Read the model definition and answer for the solid it produces. Units are mm, in the model's axes. Face numbers are marked on the shaded views. A direction names the side the tool comes from. Coordinates: 2 decimals unless noted, no trailing zeros. Order: outer loops, then holes, each group sorted by start corner. A loop starts at its lowest first (then second) coordinate and runs counter-clockwise, first axis right, second up. Notation, with made-up numbers: M -22.75,66.25 L 6.25,66.25 A12 cw 6.25,89.25 Z; hole C -39.75,57.5 d9. An arc over 180 degrees is marked long. Write each question's results on one line, items separated by ' | '.
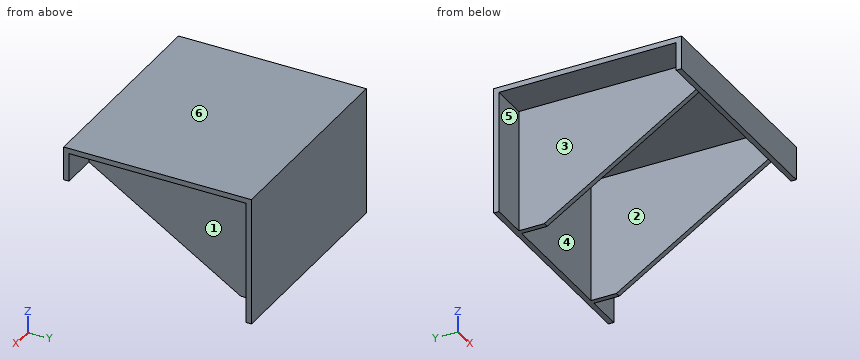
```python
from build123d import *

# Parameters (mm, degrees)
F0_W     = 320.675
F0_H     = 192.913
F1_DEPTH = 7.9375
F4_DEPTH = 266.7
F6_DEPTH = 265.1135
F8_W     = 320.675
F8_H     = 50.8
F9_DEPTH = 7.9375


with BuildPart() as f1:
    # F0 (on Front) → F1 (new body)
    with BuildSketch(Plane.XZ):
        with Locations((0, -96.4565)):
            Rectangle(F0_W, F0_H)
    extrude(amount=F1_DEPTH)

    # F3 (on face) → F4 (join)
    with BuildSketch(Plane.XZ.offset(7.9375)):
        Polygon((160.3375, 0), (-160.3375, 0), (-160.3375, -7.9375), (-104.775, -7.9375), (-104.775, -192.913), (-96.8375, -192.913), (-96.8375, -7.9375), (96.8375, -7.9375), (96.8375, -192.913), (104.775, -192.913), (104.775, -7.9375), (160.3375, -7.9375), align=None)
    extrude(amount=F4_DEPTH)

    # F5 (on face) → F6 (cut, through all)
    with BuildSketch(Plane(origin=(-104.775, 0, 0), x_dir=(0, -1, 0), z_dir=(-1, 0, 0))):
        Polygon((274.6375, -50.8), (46.0375, -192.913), (274.6375, -192.913), align=None)
    extrude(amount=-F6_DEPTH, mode=Mode.SUBTRACT)

    # F8 (on face) → F9 (join)
    with BuildSketch(Plane.XZ.offset(274.6375)):
        with Locations((0, -25.4)):
            Rectangle(F8_W, F8_H)
    extrude(amount=F9_DEPTH)


solid = f1.part
```
(1) The part is cut by section A-A, the plane z = -38.5. Write down the section's boundary in (x, y) (1 decimal), then the cut area to 3 significant figures.
Conclusion:
outline: M -160.3,-282.6 L 160.3,-282.6 L 160.3,-274.6 L 104.8,-274.6 L 104.8,-7.9 L 160.3,-7.9 L 160.3,0 L -160.3,0 L -160.3,-7.9 L -104.8,-7.9 L -104.8,-274.6 L -160.3,-274.6 Z; hole M -96.8,-274.6 L 96.8,-274.6 L 96.8,-7.9 L -96.8,-7.9 Z | area: 9,320 mm²
(2) Straight lines are drawn through the part: line 1 (X direction, y = -135.5, z = -32) (1 decimal); line 2 (Y direction, x = -109.5, z = -12.5) (1 decimal); line 3 (Y direction, x = 94.5, z = -53.5). For each, find the intervals that lie inside material, in ascending order.
Conclusion:
line 1: -104.8 to -96.8, 96.8 to 104.8 | line 2: -282.6 to -274.6, -7.9 to 0 | line 3: -7.94 to 0
(3) The part is cut by section D-D, the plane z = -181. Write down the section's boundary in (x, y) (1 decimal), then the cut area to 3 significant figures.
Conclusion:
outline: M -160.3,-7.9 L -104.8,-7.9 L -104.8,-65.2 L -96.8,-65.2 L -96.8,-7.9 L 96.8,-7.9 L 96.8,-65.2 L 104.8,-65.2 L 104.8,-7.9 L 160.3,-7.9 L 160.3,0 L -160.3,0 Z | area: 3,450 mm²
(4) The part is cut by section B-B, the plane x = 20. Write down the section's boundary in (y, z) (1 decimal).
Conclusion:
outline: M -282.6,-50.8 L -274.6,-50.8 L -274.6,-7.9 L -7.9,-7.9 L -7.9,-192.9 L 0,-192.9 L 0,0 L -282.6,0 Z
(5) The part is cut by section C-C, the plane y = -32.5. Write down the section's boundary in (x, z) (1 decimal).
Conclusion:
outline: M -160.3,-7.9 L -104.8,-7.9 L -104.8,-192.9 L -96.8,-192.9 L -96.8,-7.9 L 96.8,-7.9 L 96.8,-192.9 L 104.8,-192.9 L 104.8,-7.9 L 160.3,-7.9 L 160.3,0 L -160.3,0 Z
(6) The mould has two halves that part along X. Classify the marked faces 1, 2 and 3: pulls with the +X half, pulls with the -X half, needs draft (parallel to the pull), parting line crosses it, or undercut.
Conclusion:
face 1: pulls with the +X half | face 2: undercut | face 3: pulls with the -X half
(7) Given pin 1 (5 mm diameter, centred on y = -139.5, z = -122.5, fed in from -X) (3 decimals); pin 2 (4 mm diameter, centred on y = -60.5, z = -32, fed in from +X) (3 decimals); pin 3 (1 mm diameter, centred on x = 71, z = -159, fed in from -Y), each flat-ended and moving along its own axis, determine where each tip first touches the part or whether it passes through.
Conclusion:
pin 1: x = -104.775 | pin 2: x = 104.775 | pin 3: y = -7.94
(8) For the marked faces 4, 5 and 6, determine the directions among +Z, -Z, +X, -X, +Y, -Y from which every point of the face is accessible in a straight line to the end or side of a thin tool.
Conclusion:
face 4: -Z | face 5: -Z, -X | face 6: +Z, +X, -X, +Y, -Y
